Part model, mm, in its own coordinate system. Face numbers are marked on the shaded views. A direction names the side the tool comes from. Round coordinates to 2 decimals unless told otherwise and drop trailing zeros. Write each loop counter-clockwise with the first axis right and the second up, starting at its lowest first coordinate (ties: lowest second). Pieces come first, ordered by that corner, then holes.
from build123d import *

# Parameters (mm, degrees)
SKETCH_1_W          = 20
SKETCH_1_H          = 13
SKETCH_1_R          = 1.6
EXTRUDE_1_DEPTH     = 3
SKETCH_2_W          = 3
SKETCH_2_H          = 13
EXTRUDE_2_DEPTH     = 31
SKETCH_3_R          = 4.13
CUT_EXTRUDE_1_DEPTH = 1.5
CUT_EXTRUDE_2_DEPTH = 10
FILLET_1_R          = 2


with BuildPart() as part:
    # 草图1 → 凸台-拉伸1 (new body)
    with BuildSketch(Plane(origin=(0, 0, 0), x_dir=(1, 0, 0), z_dir=(0, 1, 0))):
        Rectangle(SKETCH_1_W, SKETCH_1_H)
        with Locations(Location((0, 3, 0), (0, 0, 270))):
            Circle(SKETCH_1_R, mode=Mode.SUBTRACT)
        with Locations(Location((3, 0, 0), (0, 0, 270))):
            Circle(SKETCH_1_R, mode=Mode.SUBTRACT)
        with Locations(Location((0, -3, 0), (0, 0, 90))):
            Circle(SKETCH_1_R, mode=Mode.SUBTRACT)
        with Locations(Location((-3, 0, 0), (0, 0, 90))):
            Circle(SKETCH_1_R, mode=Mode.SUBTRACT)
    extrude(amount=EXTRUDE_1_DEPTH)

    # 草图2 → 凸台-拉伸2 (add)
    with BuildSketch(Plane(origin=(0, 0, 0), x_dir=(1, 0, 0), z_dir=(0, 1, 0))):
        with Locations((11.5, 0)):
            Rectangle(SKETCH_2_W, SKETCH_2_H)
        with Locations((-11.5, 0)):
            Rectangle(SKETCH_2_W, SKETCH_2_H)
    extrude(amount=EXTRUDE_2_DEPTH)

    # 草图3 → 切除-拉伸1 (cut)
    with BuildSketch(Plane.ZY.offset(-10)):
        with Locations((0, 24)):
            Circle(SKETCH_3_R)
    extrude(amount=-CUT_EXTRUDE_1_DEPTH, mode=Mode.SUBTRACT)

    # 草图4 → 切除-拉伸2 (cut)
    with BuildSketch(Plane(origin=(-10, 0, 0), x_dir=(0, 0, -1), z_dir=(1, 0, 0))):
        with BuildLine():
            Line((1.526302722, 25.8), (-1.526302722, 25.8))
            ThreePointArc((-1.526302722, 25.8), (-2.36, 24), (-1.526302722, 22.2))
            Line((-1.526302722, 22.2), (1.526302722, 22.2))
            ThreePointArc((1.526302722, 22.2), (2.36, 24), (1.526302722, 25.8))
        make_face()
    extrude(amount=-CUT_EXTRUDE_2_DEPTH, mode=Mode.SUBTRACT)

    # 圆角1
    fillet_1_edges = [part.edges().sort_by_distance(p)[0] for p in [
        (-11.5, 31, -6.5),
        (-11.5, 31, 6.5),
        (11.5, 31, 6.5),
        (11.5, 31, -6.5),
    ]]
    fillet(fillet_1_edges, radius=FILLET_1_R)


solid = part.part
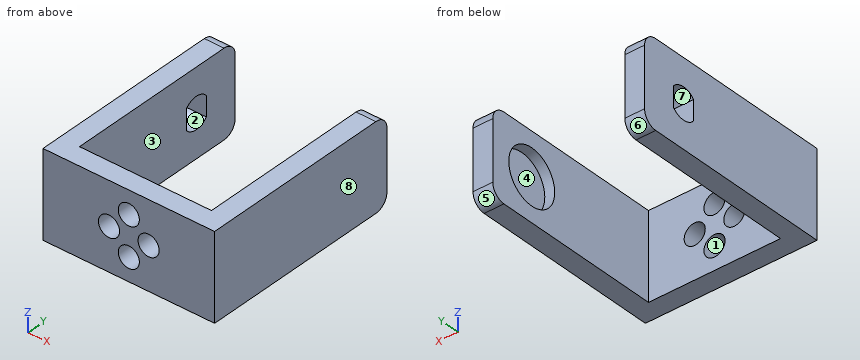
Q1. Saw through at B-B, the plane x = 0. Write the cut outline in (y, z).
Q2. Two-plate mould, pull along Y, no slides. Class the marked faces 6, 7 and 8: released by +Y, released by -Y, zero draft, split by the parting line, or undercut.
Q3. Saw through at D-D, the plane x = -3. Write the cut outline in (y, z), and give its area (3 significant figures).
Q4. Saw through at C-C, the plane y = 24. Write the cut outline in (x, z), and give its area (4 significant figures).
Q5. Drop flat-ended pins along their axis: P1, Ø2.5, axis at x = 3, z = 0, coming from the +Y side; P2, Ø5, axis at x = 4.5, z = 1, coming from the +Y side. Give the stop position or say it passes through.
Q6. Wall check: line 1 (X direction, y = 15, z = 3.5); line 2 (X direction, y = 1.95, z = -3); line 3 (Y direction, x = 10.5, z = 0). Give the ranges that are in metal, low to high.
Q7. Tool access for the marked faces 1, 2, 3, 4 and 5: list every direction of +Z, -Z, +X, -X, +Y, -Y with a clear straight run to the whole face (end or side of a thin tool).
Q8. Saw through at A-A, the plane z = 0. Write the cut outline in (x, y).
Computed:
1. outline: (0, -6.5) - (3, -6.5) - (3, -4.6) - (0, -4.6) - close; (0, -1.4) - (3, -1.4) - (3, 1.4) - (0, 1.4) - close; (0, 4.6) - (3, 4.6) - (3, 6.5) - (0, 6.5) - close
2. face 6: released by +Y
2. face 7: undercut
2. face 8: zero draft
3. outline: (0, -6.5) - (3, -6.5) - (3, -1.6) - (0, -1.6) - close; (0, 1.6) - (3, 1.6) - (3, 6.5) - (0, 6.5) - close
3. area: 29.4 mm2
4. outline: (-13, -6.5) - (-10, -6.5) - (-10, -2.36) - (-13, -2.36) - close; (-13, 2.36) - (-10, 2.36) - (-10, 6.5) - (-13, 6.5) - close; (10, -6.5) - (13, -6.5) - (13, 6.5) - (10, 6.5) - (10, 4.13) - (11.5, 4.13) - (11.5, -4.13) - (10, -4.13) - close
4. area: 51.45 mm2
5. P1: passes through
5. P2: stops at y = 3
6. line 1: x = -13 to -10, 10 to 13
6. line 2: x = -13 to -1.6, 1.6 to 13
6. line 3: y = 0 to 19.87, 28.13 to 31
7. face 1: +Y, -Y
7. face 2: -X
7. face 3: +Z, -Z, +Y
7. face 4: none
7. face 5: -Z, +X, -X, +Y
8. outline: (-13, 0) - (-4.6, 0) - (-4.6, 3) - (-10, 3) - (-10, 22.2) - (-13, 22.2) - close; (-13, 25.8) - (-10, 25.8) - (-10, 31) - (-13, 31) - close; (-1.4, 0) - (1.4, 0) - (1.4, 3) - (-1.4, 3) - close; (4.6, 0) - (13, 0) - (13, 31) - (10, 31) - (10, 28.13) - (11.5, 28.13) - (11.5, 19.87) - (10, 19.87) - (10, 3) - (4.6, 3) - close
